from build123d import *

# Parameters (mm, degrees)
F0_W         = 20
F0_H         = 60
F0_R         = 4
F0_R_2       = 6.25
F1_DEPTH     = 4
F1_FACE_W    = 20
F1_FACE_H    = 60
F1_FACE_R    = 4
F1_FACE_R_2  = 6.25
F0_R_3       = 2.75
F2_DEPTH     = 1
F3_W         = 5
F3_H         = 5
F4_DEPTH     = 5
F5_T1_DEPTH  = 97.9025398997
F6_R         = 2.49999
F7_R         = 1.1
F8_DEPTH     = 25
F9_DEPTH     = 5
F10_T1_DEPTH = 97.8518303197
F11_DEPTH    = 2


# Not quite as in the source:
# - a fillet or chamfer that OpenCascade refuses, or shapes differently, is made with other operations: its cross-section is extruded or revolved along the edge and cut away or added
# - a fillet or chamfer is up to 0.001 mm smaller than in the source, because OpenCascade refuses the exact size


with BuildPart() as f1:
    # F0 (on Top) → F1 (new body)
    with BuildSketch(Plane.XY):
        with Locations((10, 30)):
            Rectangle(F0_W, F0_H)
        with Locations((10, 10)):
            Circle(F0_R, mode=Mode.SUBTRACT)
        with Locations((10, 40)):
            Circle(F0_R_2, mode=Mode.SUBTRACT)
    extrude(amount=F1_DEPTH)

    # F1_face (on face) + F0 (on Top) → F2 (join)
    with BuildSketch(Plane(origin=(10, 29.783961526, 4), x_dir=(1, 0, 0), z_dir=(0, 0, 1))):
        with Locations((0, 0.216038474)):
            Rectangle(F1_FACE_W, F1_FACE_H)
        with Locations((0, -19.783961526)):
            Circle(F1_FACE_R, mode=Mode.SUBTRACT)
        with Locations((0, 10.216038474)):
            Circle(F1_FACE_R_2, mode=Mode.SUBTRACT)
    with BuildSketch(Plane.XY):
        with Locations((10, 10)):
            Circle(F0_R)
        with Locations((10, 10)):
            Circle(F0_R_3, mode=Mode.SUBTRACT)
    extrude(amount=F2_DEPTH)

    # F3 (on face) → F4 (join)
    with BuildSketch(Plane.XY.offset(5)):
        with Locations((2.5, 17.5)):
            Rectangle(F3_W, F3_H)
        with Locations((17.5, 17.5)):
            Rectangle(F3_W, F3_H)
    extrude(amount=F4_DEPTH)

    # F5: chamfer of 15 x 4 on 1 edges, made by hand

    # F5_s2 → F5_t1 (cut)
    with BuildSketch(Plane.YZ.offset(-38.9512699498)):
        Polygon((15, 5), (0, 1), (0, 5), align=None)
    extrude(amount=F5_T1_DEPTH, mode=Mode.SUBTRACT)

    # F6 (radius 2.5 in the source; OpenCascade refuses exactly that, so slightly less here)
    f6_edges = [f1.edges().sort_by_distance(p)[0] for p in [
        (2.5, 15, 5),
        (2.5, 15, 10),
        (17.5, 15, 5),
        (17.5, 15, 10),
        (2.5, 20, 10),
        (17.5, 20, 10),
    ]]
    fillet(f6_edges, radius=F6_R)

    # F7 (on face) → F8 (cut)
    with BuildSketch(Plane(origin=(0, 0, 0), x_dir=(0, -1, 0), z_dir=(-1, 0, 0))):
        with Locations((-17.5, 7.5)):
            Circle(F7_R)
    extrude(amount=-F8_DEPTH, mode=Mode.SUBTRACT)

    # F10: chamfer of 5 x 15 on 1 edges, made by hand

    # F10_s2 → F10_t1 (cut)
    with BuildSketch(Plane.YZ.offset(-38.9259151598)):
        Polygon((60, 0), (45, 5), (60, 5), align=None)
    extrude(amount=F10_T1_DEPTH, mode=Mode.SUBTRACT)



with BuildPart() as f9:
    # F0 (on Top) → F9 (new body)
    with BuildSketch(Plane.XY):
        with Locations((10, 10)):
            Circle(F0_R)
        with Locations((10, 10)):
            Circle(F0_R_3, mode=Mode.SUBTRACT)
    extrude(amount=F9_DEPTH)


with BuildPart() as f1_1:
    add(f1.part)

    add(f9.part)  # F11 merges F9
    # F0 (on Top) → F11 (join)
    with BuildSketch(Plane.XY):
        with Locations((10, 10)):
            Circle(F0_R_3)
    extrude(amount=F11_DEPTH)


solid = f1_1.part
Design review of the part built by this model. Coordinates are the model's own, in mm. A direction names the side the tool comes from. Give positions to 0.01 mm unless a question says otherwise; leave off trailing zeros. Loops run counter-clockwise (first coordinate to the right, second up) from the corner with the lowest first, then second, coordinate; pieces in that order, holes last. Notation, with made-up numbers: (-30.75, 35) - (-3.75, 35) arc R17 cw to (-3.75, 55) - close; hole circle Ø5 at (30.5, 26.5). An arc over 180 degrees is marked (long way). Use CSV: the item, a comma, the result in double quotes. Start each with the question number.
1. Add section B-B (x = 8.5). State the section outline as (y, z) points, plus the area to 3 significant figures.
2. Machinability: for faces 1 (the flat face through (17, 20, 6)), 2 (the cylindrical face through (17.535, 15.713, 9.248)), 3 (the cylindrical face through (17.54, 14.47, 5.38)), which of the approach directions +Z, -Z, +X, -X, +Y, -Y give a long, thin tool a straight path to every point of the face, cutting with its end or side? Answer none if there is none.
3. Add section C-C (x = 11.25). State the section outline as (y, z) points.
4. Insertion check: P1, Ø6, axis at x = 11, y = 9, coming from the +Z side; P2, Ø0.8, axis at x = 18.5, z = 6.5, coming from the +Y side. Each pin has a flat end and moves straight along its axis. Give the tip position at first contact, or say it passes through.
5. Add section A-A (y = 40). State the section outline as (x, z) points, plus the area to 3 significant figures.
6. Wall thickness on L1, parallel to X at y = 40, z = 2.7; L2, parallel to Z at x = 18.3, y = 17.5; L3, parallel to X at y = 17.5, z = 5.5: over which ranges is each line inside the solid? List them lowest first.
7. Draft analysis for pull direction Z (two halves, no side actions). For faces 4 (the flat face through (12.082, 5.938, 2.584)), 5 (the cylindrical face through (11.48, 12.32, 3.48)), 6 (the flat face through (10, 30, 0)), 7 (the cylindrical face through (17.5, 18.6, 7.5)), state which applies: released by +Z, released by -Z, zero draft, split by the parting line, or undercut.
Results found:
1,outline,"(0, 0) - (33.93, 0) - (33.93, 5) - (15, 5) - (13.71, 4.66) - (13.71, 5) - (12.3, 5) - (12.3, 2) - (7.7, 2) - (7.7, 5) - (6.29, 5) - (6.29, 2.68) - (0, 1) - close; (46.07, 0) - (60, 0) - (46.07, 4.64) - close"
1,area,"168 mm²"
2,face 1,"+Z, +X, -X, +Y"
2,face 2,"+Z, +X, -X, -Y"
2,face 3,"+Z, +X, -Y"
3,outline,"(0, 0) - (33.88, 0) - (33.88, 5) - (15, 5) - (13.8, 4.68) - (13.8, 5) - (12.45, 5) - (12.45, 2) - (7.55, 2) - (7.55, 5) - (6.2, 5) - (6.2, 2.65) - (0, 1) - close; (46.12, 0) - (60, 0) - (46.12, 4.63) - close"
4,P1,"stops at z = 5"
4,P2,"stops at y = 20"
5,outline,"(0, 0) - (3.75, 0) - (3.75, 5) - (0, 5) - close; (16.25, 0) - (20, 0) - (20, 5) - (16.25, 5) - close"
5,area,"37.5 mm²"
6,L1,"x = 0 to 3.75, 16.25 to 20"
6,L2,"z = 0 to 6.4, 8.6 to 10"
6,L3,"x = 0 to 5, 15 to 20"
7,face 4,"released by +Z"
7,face 5,"zero draft"
7,face 6,"released by -Z"
7,face 7,"undercut"
